Check sheet for the modelled part. Datum: model origin and axes. Units: mm. A direction names the side the tool comes from. Round coordinates to 2 decimals unless told otherwise and drop trailing zeros. Loops run counter-clockwise (first coordinate to the right, second up) from the corner with the lowest first, then second, coordinate; pieces in that order, holes last. Notation, with made-up numbers: (68, 66.25) - (92, 66.25) arc R26 cw to (92, 91.25) - close; hole circle Ø3 at (18, 44.5). An arc over 180 degrees is marked (long way). Put each result on its own line as item: value. Start each with the question number.
Item 1: Tool access check on faces 1 (the flat face through (1, -2.54, 3)), 2 (the flat face through (0, 0, 0)), 3 (the cylindrical face through (-2.52, -18.87, -1.93)). Record the directions out of +Z, -Z, +X, -X, +Y, -Y that give a thin tool (end or side, any length) a straight path to the whole face; none if there is none.
Item 2: Section check A-A, the plane z = 0. Record the cut outline in (x, y), and give its area (3 significant figures).
Item 3: Section check B-B, the plane x = -1.25. Record the cut outline in (y, z).
Item 4: Gauge pin test, flat ends, axial feed: pin 1 Ø2 at (x, y) = (3.5, -8.5) entering from +Z; pin 2 Ø2 at (y, z) = (-28.5, 3) entering from -X; pin 3 Ø4 at (y, z) = (-6, 4) entering from -X. Record the tip position at first contact, or that the pin passes through.
Item 5: Material ranges on line 1 along Y through (x, z) = (-2.5, -3); line 2 along Y through (x, z) = (0.5, 3.5); line 3 along X through (y, z) = (-10.5, -2.25), recorded low to high.
Item 6: Section check D-D, the plane y = -6. Record the cut outline in (x, z).
Item 7: Draft check along Z on faces 4 (the cylindrical face through (-5.029, -3.131, -3.856)), 5 (the cylindrical face through (0.98, -1.25, 1.56)), 6 (the flat face through (0, -31.75, 0)). Enter one of: pulls with the +Z half, pulls with the -Z half, needs draft (parallel to the pull), parting line crosses it, or undercut.
Item 8: Section check C-C, the plane y = -21.5. Record the cut outline in (x, z).
from build123d import *

# Parameters (mm, degrees)
F0_R     = 6.3373
F1_DEPTH = 6.35
F2_R     = 3.17373
F3_DEPTH = 25.4
F4_R     = 1.5875
F5_DEPTH = 2.54


with BuildPart() as f1:
    # F0 (on Front) → F1 (new body)
    with BuildSketch(Plane.XZ):
        Circle(F0_R)
    extrude(amount=F1_DEPTH)

    # F2 (on face) → F3 (join)
    with BuildSketch(Plane.XZ.offset(6.35)):
        Circle(F2_R)
    extrude(amount=F3_DEPTH)

    # F4 (on face) → F5 (cut)
    with BuildSketch(Plane(origin=(0, 0, 0), x_dir=(-1, 0, 0), z_dir=(0, 1, 0))):
        with Locations((-0.635, 3.110852)):
            Circle(F4_R)
    extrude(amount=-F5_DEPTH, mode=Mode.SUBTRACT)


solid = f1.part
Check result:
1. face 1: +Y
1. face 2: +Z, -Z, +X, -X, +Y
1. face 3: -Y
2. outline: (-6.34, -6.35) - (-3.17, -6.35) - (-3.17, -31.75) - (3.17, -31.75) - (3.17, -6.35) - (6.34, -6.35) - (6.34, 0) - (-6.34, 0) - close
2. area: 242 mm²
3. outline: (-31.75, -2.92) - (-6.35, -2.92) - (-6.35, -6.21) - (0, -6.21) - (0, 6.21) - (-6.35, 6.21) - (-6.35, 2.92) - (-31.75, 2.92) - close
4. pin 1: z = 1.96
4. pin 2: x = -2.46
4. pin 3: x = -6.01
5. line 1: -6.35 to 0
5. line 2: -6.35 to -2.54
5. line 3: -2.24 to 2.24
6. outline: circle Ø12.67 at (0, 0)
7. face 4: parting line crosses it
7. face 5: undercut
7. face 6: needs draft
8. outline: circle Ø6.35 at (0, 0)
